Input: part model. Units: mm. Frame: model coordinates. A direction names the side the tool comes from. Give positions to 0.01 mm unless a question says otherwise; leave off trailing zeros. Loops run counter-clockwise (first coordinate to the right, second up) from the corner with the lowest first, then second, coordinate; pieces in that order, holes last. Notation, with made-up numbers: (84.5, 0) -> (88.5, 0) arc R35 cw to (88.5, 39) -> close; hole circle Ø1 at (80.25, 54). An arc over 180 degrees is marked (long way). Answer as a JSON object with one key per item and string values.
```python
from build123d import *

# Parameters (mm, degrees)
SALIENTE_EXTRUIR1_DEPTH = 5
CROQUIS6_R              = 6
SALIENTE_EXTRUIR2_DEPTH = 5
EXTRUIR_L_MINA1_DEPTH   = 5
CROQUIS9_R              = 12.5
CROQUIS9_R_2            = 7.5
SALIENTE_EXTRUIR3_DEPTH = 18
CROQUIS10_R             = 15
SALIENTE_EXTRUIR4_DEPTH = 5
CROQUIS10_3_R           = 12.5
SALIENTE_EXTRUIR5_DEPTH = 10
CROQUIS11_R             = 7.5
CORTAR_EXTRUIR1_DEPTH   = 20


# Read off the part's stored shape, not the designer's step: Extruir-Lámina1
with BuildPart() as part:
    # Croquis1 → Saliente-Extruir1 (new, symmetric)
    with BuildSketch(Plane(origin=(0, 0, 0), x_dir=(1, 0, 0), z_dir=(0, 1, 0))):
        with BuildLine():
            Line((-135, 131.926889983), (-105, 131.926889983))
            Line((-105, 131.926889983), (-97.355197186, 120.822380101))
            ThreePointArc((-97.355197186, 120.822380101), (-91.978989417, 116.050643627), (-85, 114.328207662))
            Line((-85, 114.328207662), (85, 114.328207662))
            ThreePointArc((85, 114.328207662), (91.978989417, 116.050643627), (97.355197186, 120.822380101))
            Line((97.355197186, 120.822380101), (105, 131.926889983))
            Line((105, 131.926889983), (135, 131.926889983))
            add(Edge.make_bspline(
                [(135, 131.926889983), (141.952707227, 30.351328575), (23.130947771, -13.752661754), (25, -115)],
                knots=[0, 0, 0, 0, 1, 1, 1, 1], degree=3))
            ThreePointArc((25, -115), (0, -140), (-25, -115))
            add(Edge.make_bspline(
                [(-135, 131.926889983), (-141.952707227, 30.351328575), (-23.130947771, -13.752661754), (-25, -115)],
                knots=[0, 0, 0, 0, 1, 1, 1, 1], degree=3))
        make_face()
        with BuildLine():
            Line((-67.388374008, 41.875089785), (-11.082561012, -19.857874005))
            ThreePointArc((-11.082561012, -19.857874005), (0, -24.749617904), (11.082561012, -19.857874005))
            Line((11.082561012, -19.857874005), (67.388374008, 41.875089785))
            ThreePointArc((67.388374008, 41.875089785), (69.148452711, 52.651972876), (60, 58.613927185))
            Line((60, 58.613927185), (-60, 58.613927185))
            ThreePointArc((-60, 58.613927185), (-69.148452711, 52.651972876), (-67.388374008, 41.875089785))
        make_face(mode=Mode.SUBTRACT)
    extrude(amount=SALIENTE_EXTRUIR1_DEPTH, both=True)

    # Croquis6 → Saliente-Extruir2 (add)
    with BuildSketch(Plane(origin=(5, 0, 0), x_dir=(0, 0, -1), z_dir=(1, 0, 0))):
        with BuildLine():
            Line((-34.749617904, 5), (-54.446317045, 24.696699141))
            ThreePointArc((-54.446317045, 24.696699141), (-59.749617904, 26.893398282), (-65.052918763, 24.696699141))
            Line((-65.052918763, 24.696699141), (-84.749617904, 5))
            Line((-84.749617904, 5), (-34.749617904, 5))
        make_face()
        with Locations((-59.749617904, 14.393398282)):
            Circle(CROQUIS6_R, mode=Mode.SUBTRACT)
    saliente_extruir2 = extrude(amount=SALIENTE_EXTRUIR2_DEPTH)

    # Simetría1: Saliente-Extruir2 across plane
    add(saliente_extruir2.mirror(Plane(origin=(0, 0, 0), x_dir=(0, 0, 1), z_dir=(1, 0, 0))))

    # Extruir-Lámina1 outline → Extruir-Lámina1 (add)
    with BuildSketch(Plane(origin=(0, 5, 0), x_dir=(1, 0, 0), z_dir=(0, 1, 0))):
        with BuildLine():
            Line((-106.051245454, 129.926889983), (-133.152785768, 129.926889983))
            add(Edge.make_bspline(
                [(-133.152785768, 129.926889983), (-133.174268661, 129.206657548), (-133.195751554, 128.486425113), (-133.238717339, 127.045960243), (-133.260373261, 126.325704896), (-133.29971078, 124.168332797), (-133.301445055, 119.863777053), (-133.071902544, 115.589846855), (-132.303121335, 107.08299626), (-131.375659828, 101.466708751), (-129.377010697, 93.122716596), (-128.609455105, 90.354805161), (-127.310297322, 86.222512835), (-126.853085806, 84.849889782), (-125.898422992, 82.13221094), (-125.400190812, 80.784491049), (-122.810267538, 74.098434679), (-120.42291954, 68.917392178), (-115.158069426, 58.816076633), (-112.280987066, 53.895580273), (-107.696886081, 46.657669825), (-106.124147998, 44.268816441), (-102.905009703, 39.53029905), (-101.257661562, 37.179322504), (-92.887901697, 25.518907347), (-85.780126078, 16.499131041), (-71.58045013, -1.552311855), (-64.485262059, -10.58151599), (-56.133776454, -22.255618212), (-54.489378689, -24.60983677), (-51.266448327, -29.367605618), (-49.686457, -31.773531765), (-45.084200101, -39.052900232), (-42.196352007, -43.992840655), (-36.899381702, -54.103765632), (-34.490320683, -59.274779718), (-31.324385536, -67.247350119), (-30.343694104, -69.940887052), (-28.995690401, -74.040571223), (-28.566659059, -75.417806864), (-27.752342999, -78.1897194), (-27.36871345, -79.578876355), (-25.569409892, -86.540828042), (-24.511463015, -92.162286021), (-23.173842405, -103.511074009), (-22.89542751, -109.238575264), (-22.999992819, -115.018175056)],
                knots=[0, 0, 0, 0, 0.0078125, 0.0078125, 0.015625, 0.015625, 0.03125, 0.0625, 0.0625, 0.125, 0.125, 0.15625, 0.15625, 0.171875, 0.171875, 0.1875, 0.1875, 0.25, 0.25, 0.3125, 0.3125, 0.34375, 0.34375, 0.375, 0.375, 0.5, 0.5, 0.625, 0.625, 0.65625, 0.65625, 0.6875, 0.6875, 0.75, 0.75, 0.8125, 0.8125, 0.84375, 0.84375, 0.859375, 0.859375, 0.875, 0.875, 0.9375, 0.9375, 1, 1, 1, 1], degree=3))
            ThreePointArc((-22.999992819, -115.018175056), (0, -138), (22.999992819, -115.018175056))
            add(Edge.make_bspline(
                [(22.999992819, -115.018175056), (22.895226578, -109.227469196), (23.175119897, -103.499493799), (24.510635399, -92.170049231), (25.564939035, -86.568365032), (27.708902858, -78.257572863), (28.51704955, -75.502555539), (29.865517568, -71.392248939), (30.338548889, -70.023401781), (31.323606713, -67.307934522), (33.883396821, -60.573683364), (36.902914511, -54.096952925), (44.842899172, -38.941069981), (51.05964732, -29.354413219), (59.399269025, -17.689647357), (61.096404781, -15.371876329), (64.528507919, -10.767382329), (66.263972325, -8.479913942), (71.509332424, -1.647173505), (75.058209766, 2.868422579), (82.159416645, 11.896986658), (85.711763576, 16.409941411), (92.71853999, 25.510393556), (96.172818384, 30.098005967), (101.199601756, 37.097144589), (102.850583686, 39.451755912), (106.077537799, 44.198688655), (107.653878795, 46.591420768), (112.247661329, 53.839778233), (115.129622576, 58.765689131), (120.401963318, 68.872537636), (122.791888775, 74.053710792), (125.900918311, 82.072340278), (126.85794185, 84.78636685), (128.595390264, 90.306037259), (129.365828105, 93.080127996), (131.371298301, 101.438867894), (132.300684578, 107.06336018), (133.071299421, 115.579637461), (133.224668995, 118.431600887), (133.300279497, 122.729249291), (133.29974204, 124.165082676), (133.260423161, 126.323746033), (133.238764128, 127.044391606), (133.195774948, 128.485640795), (133.174280358, 129.206265389), (133.152785768, 129.926889983)],
                knots=[0, 0, 0, 0, 0.0625, 0.0625, 0.125, 0.125, 0.15625, 0.15625, 0.171875, 0.171875, 0.1875, 0.25, 0.25, 0.375, 0.375, 0.40625, 0.40625, 0.4375, 0.4375, 0.5, 0.5, 0.5625, 0.5625, 0.625, 0.625, 0.65625, 0.65625, 0.6875, 0.6875, 0.75, 0.75, 0.8125, 0.8125, 0.84375, 0.84375, 0.875, 0.875, 0.9375, 0.9375, 0.96875, 0.96875, 0.984375, 0.984375, 0.9921875, 0.9921875, 1, 1, 1, 1], degree=3))
            Line((133.152785768, 129.926889983), (106.051245454, 129.926889983))
            Line((106.051245454, 129.926889983), (99.00255681, 119.688269759))
            ThreePointArc((99.00255681, 119.688269759), (92.90952134, 114.280301755), (85, 112.328207662))
            Line((85, 112.328207662), (-85, 112.328207662))
            ThreePointArc((-85, 112.328207662), (-92.90952134, 114.280301755), (-99.00255681, 119.688269759))
            Line((-99.00255681, 119.688269759), (-106.051245454, 129.926889983))
        make_face()
        with BuildLine():
            add(Edge.make_bspline(
                [(-130.240934691, 126.926889983), (-130.411547803, 121.206938866), (-130.167660454, 115.547790898), (-128.847873599, 104.35154298), (-127.771663621, 98.814488573), (-125.924626652, 91.966775959), (-125.530222733, 90.600900181), (-124.692269656, 87.876357749), (-124.247843704, 86.515308788), (-122.852183388, 82.470259757), (-121.837255643, 79.818705121), (-118.567479133, 71.984263185), (-116.088003331, 66.921402163), (-110.672433719, 57.039667488), (-107.736270132, 52.220831119), (-103.088325832, 45.122793633), (-101.498316815, 42.778525535), (-98.252555912, 38.12511811), (-96.597218478, 35.816635505), (-88.212586529, 24.366109238), (-81.147647458, 15.472894286), (-67.116887318, -2.387674605), (-60.14620433, -11.351391892), (-51.980786937, -22.965887821), (-50.3752326, -25.30937845), (-47.232310585, -30.047362451), (-45.695210028, -32.441712267), (-41.22621426, -39.683394316), (-38.430313516, -44.598820237), (-33.314610216, -54.657139194), (-30.994773138, -59.800015737), (-27.952783748, -67.72348367), (-27.011738958, -70.399494027), (-25.719660825, -74.470598268), (-25.308321792, -75.839168342), (-24.529959844, -78.586079762), (-24.163389081, -79.962558454), (-22.44464198, -86.860207974), (-21.435659553, -92.427263793), (-20.161720093, -103.660851552), (-19.89654276, -109.327354037), (-19.999953481, -115.043136709)],
                knots=[0, 0, 0, 0, 0.0625, 0.0625, 0.125, 0.125, 0.140625, 0.140625, 0.15625, 0.15625, 0.1875, 0.1875, 0.25, 0.25, 0.3125, 0.3125, 0.34375, 0.34375, 0.375, 0.375, 0.5, 0.5, 0.625, 0.625, 0.65625, 0.65625, 0.6875, 0.6875, 0.75, 0.75, 0.8125, 0.8125, 0.84375, 0.84375, 0.859375, 0.859375, 0.875, 0.875, 0.9375, 0.9375, 1, 1, 1, 1], degree=3))
            Line((-130.240934691, 126.926889983), (-107.628113635, 126.926889983))
            Line((-107.628113635, 126.926889983), (-101.473596247, 117.987104247))
            ThreePointArc((-101.473596247, 117.987104247), (-94.305319223, 111.624788948), (-85, 109.328207662))
            Line((-85, 109.328207662), (85, 109.328207662))
            ThreePointArc((85, 109.328207662), (94.305319223, 111.624788948), (101.473596247, 117.987104247))
            Line((101.473596247, 117.987104247), (107.628113635, 126.926889983))
            Line((107.628113635, 126.926889983), (130.240934691, 126.926889983))
            add(Edge.make_bspline(
                [(19.999953481, -115.043136709), (19.896427023, -109.32095693), (20.162471748, -103.656694634), (21.433484981, -92.443970754), (22.438644162, -86.895539052), (24.487167219, -78.657640706), (25.259980416, -75.925774614), (26.550800135, -71.848599206), (27.003831738, -70.490678553), (27.947611297, -67.796645784), (28.438448915, -66.459946369), (30.982768295, -59.825525168), (33.30643755, -54.67491864), (40.970707434, -39.600575574), (47.003894339, -30.053947563), (55.153034009, -18.451527139), (56.813969399, -16.146756985), (60.17676541, -11.571661263), (65.284475951, -4.757529312), (70.527406248, 1.95332666), (77.541655616, 10.883052022), (81.060774666, 15.338753839), (88.025039956, 24.30665524), (91.470366291, 28.818717273), (96.504855219, 35.688773254), (98.16144298, 37.996989622), (101.405963711, 42.643758601), (102.99490041, 44.983639174), (107.638239543, 52.064402242), (110.569379356, 56.866302948), (118.67461083, 71.612676057), (123.164034637, 81.896076903), (126.554911876, 94.28650979), (126.908556251, 95.67466944), (127.567304158, 98.475017725), (127.87138094, 99.883309895), (128.701614509, 104.108909856), (129.147967615, 106.936415177), (130.164965006, 115.450310911), (130.412704392, 121.16816323), (130.240934691, 126.926889983)],
                knots=[0, 0, 0, 0, 0.0625, 0.0625, 0.125, 0.125, 0.15625, 0.15625, 0.171875, 0.171875, 0.1875, 0.1875, 0.25, 0.25, 0.375, 0.375, 0.40625, 0.40625, 0.4375, 0.5, 0.5, 0.5625, 0.5625, 0.625, 0.625, 0.65625, 0.65625, 0.6875, 0.6875, 0.75, 0.75, 0.875, 0.875, 0.890625, 0.890625, 0.90625, 0.90625, 0.9375, 0.9375, 1, 1, 1, 1], degree=3))
            ThreePointArc((19.999953481, -115.043136709), (0, -135), (-19.999953481, -115.043136709))
        make_face(mode=Mode.SUBTRACT)
    extrude(amount=EXTRUIR_L_MINA1_DEPTH)

    # Croquis9 → Saliente-Extruir3 (add, symmetric)
    with BuildSketch(Plane(origin=(-119.602015611, 10, -129.926889983), x_dir=(0, 0, 1), z_dir=(-1, 0, 0))):
        with Locations((-9.5, -5)):
            Circle(CROQUIS9_R)
        with Locations((-9.5, -5)):
            Circle(CROQUIS9_R_2, mode=Mode.SUBTRACT)
    saliente_extruir3 = extrude(amount=SALIENTE_EXTRUIR3_DEPTH, both=True)

    # Simetría2: Saliente-Extruir3 across plane
    add(saliente_extruir3.mirror(Plane(origin=(0, 0, 0), x_dir=(0, 0, 1), z_dir=(1, 0, 0))))

    # Croquis10 → Saliente-Extruir4 (add)
    with BuildSketch(Plane(origin=(0, 5, 0), x_dir=(1, 0, 0), z_dir=(0, 1, 0))):
        with Locations(Location((0, -115, 0), (0, 0, 90))):
            Circle(CROQUIS10_R)
    extrude(amount=SALIENTE_EXTRUIR4_DEPTH)

    # Croquis10<3> → Saliente-Extruir5 (add)
    with BuildSketch(Plane(origin=(0, 5, 0), x_dir=(1, 0, 0), z_dir=(0, 1, 0))):
        with Locations(Location((0, -115, 0), (0, 0, 270))):
            Circle(CROQUIS10_3_R)
    extrude(amount=SALIENTE_EXTRUIR5_DEPTH)

    # Croquis11 → Cortar-Extruir1 (cut)
    with BuildSketch(Plane(origin=(0, 15, 0), x_dir=(1, 0, 0), z_dir=(0, 1, 0))):
        with Locations(Location((0, -115, 0), (0, 0, 270))):
            Circle(CROQUIS11_R)
    extrude(amount=-CORTAR_EXTRUIR1_DEPTH, mode=Mode.SUBTRACT)


solid = part.part
```
Q1. Pin query (flat end, axial travel): pin 1 (10 mm diameter, centred on x = 66.5, z = -83.5, fed in from -Y); pin 2 (4 mm diameter, centred on x = 1, y = 6.5, fed in from +Z); pin 3 (2 mm diameter, centred on x = 16.5, y = -1, fed in from +Z); pin 4 (4 mm diameter, centred on x = -42.5, y = 12.5, fed in from +Z). Return the tip coordinate at first contact, or that it passes through.
Evaluation:
{"pin 1": "stops at y = -5", "pin 2": "stops at z = 140", "pin 3": "stops at z = 134.62", "pin 4": "passes through"}
Q2. Draft query along X for faces 5 (the cylindrical face through (-0.506, 7.465, 137.994)), 6 (the flat face through (137.602, -0.4, -134)), 7 (the flat face through (38.841, 0.07, -10.576)), 8 (the flat face through (-40, 10, 44)). Return one class per face: +X half, -X half, draft (parallel to the pull), parting line (faces both ways), or undercut.
Evaluation:
{"face 5": "parting line", "face 6": "+X half", "face 7": "undercut", "face 8": "draft"}
Q3. Section A-A, the plane x = 0. Return the cut outline in (y, z).
Evaluation:
{"outline": "(-5, -114.33) -> (5, -114.33) -> (5, -112.33) -> (10, -112.33) -> (10, -109.33) -> (5, -109.33) -> (5, -58.61) -> (-5, -58.61) -> close; (-5, 24.75) -> (5, 24.75) -> (5, 100) -> (10, 100) -> (10, 102.5) -> (15, 102.5) -> (15, 107.5) -> (-5, 107.5) -> close; (-5, 122.5) -> (15, 122.5) -> (15, 127.5) -> (10, 127.5) -> (10, 130) -> (5, 130) -> (5, 135) -> (10, 135) -> (10, 138) -> (5, 138) -> (5, 140) -> (-5, 140) -> close"}
Q4. Ray query, line 1 along X through (y, z) = (20.5, 68); line 2 along Y through (x, z) = (-28, -77.5); line 3 along X through (y, z) = (10.75, 115). Return the intervals inside material, ascending.
Evaluation:
{"line 1": "x = -10 to -5, 5 to 10", "line 2": "y = -5 to 5", "line 3": "x = -12.5 to -7.5, 7.5 to 12.5"}
Q5. Access query for faces 1 (the flat face through (-104.594, 7.465, -122.52)), 2 (the flat face through (34, -5, 2)), 3 (the cylindrical face through (69.213, 0.07, -52.504)), 4 (the flat face through (101.602, -0.4, -134)). Directions: +Z, -Z, +X, -X, +Y, -Y. A direction counts if a zero-diameter tool reaches every point of the face in a straight line with its end or side. Return the directions, or none.
Evaluation:
{"face 1": "+Y", "face 2": "+Z, +X, -X, -Y", "face 3": "+Y, -Y", "face 4": "-Z, +Y, -Y"}
